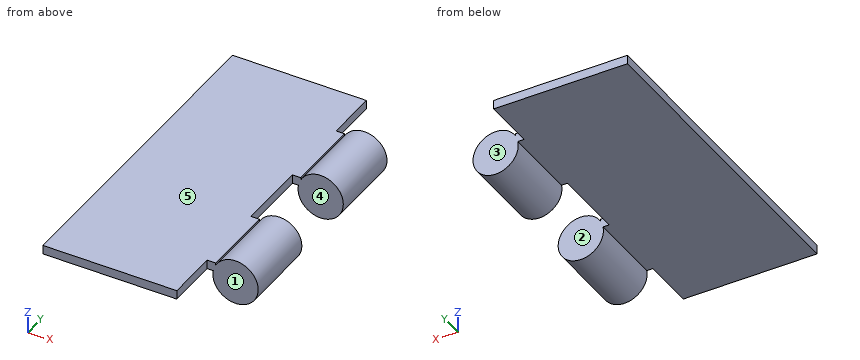
```python
from build123d import *

# Parameters (mm, degrees)
F0_W     = 31.1658
F0_H     = 76.073
F1_DEPTH = 2.0955
F2_W     = 17.526
F2_H     = 2.0955
F3_DEPTH = 1.9558
F4_R     = 5.2705
F5_DEPTH = 17.526
F7_DEPTH = 17.526


with BuildPart() as f1:
    # F0 (on Top) → F1 (new body)
    with BuildSketch(Plane.XY):
        Rectangle(F0_W, F0_H)
    extrude(amount=F1_DEPTH)

    # F2 (on face) → F3 (join)
    with BuildSketch(Plane.YZ.offset(15.5829)):
        with Locations((-17.0815, 1.04775)):
            Rectangle(F2_W, F2_H)
        with Locations((17.0815, 1.04775)):
            Rectangle(F2_W, F2_H)
    extrude(amount=F3_DEPTH)

    # F4 (on face) → F5 (join, through all)
    with BuildSketch(Plane.XZ.offset(25.8445)):
        with Locations((22.1742, -0.9652)):
            Circle(F4_R)
    extrude(amount=-F5_DEPTH)

    # F6 (on face) → F7 (join, through all)
    with BuildSketch(Plane.XZ.offset(-8.3185)):
        with BuildLine():
            Line((17.5387, 0), (16.992833, 0))
            ThreePointArc((16.992833, 0), (27.142883, -2.723141), (17.5387, 1.542849))
            Line((17.5387, 1.542849), (17.5387, 0))
        make_face()
    extrude(amount=-F7_DEPTH)


solid = f1.part
```
CAD build for the part. Positions are in the model's coordinates, mm. Face numbers are marked on the shaded views. A direction names the side the tool comes from. Round coordinates to 2 decimals unless told otherwise and drop trailing zeros. Order: outer loops, then holes, each group sorted by start corner. A loop starts at its lowest first (then second) coordinate and runs counter-clockwise, first axis right, second up. Notation, with made-up numbers: (37, 59.25) - (49, 59.25) arc R35 ccw to (49, 92.25) - close; hole circle Ø2 at (42, 88.25). An arc over 180 degrees is marked (long way). Answer as CSV lines item,"result". Start each with the question number.
1. Saw through at A-A, the plane z = -4.25. Write the cut outline in (x, y).
2. Tool access for the marked faces 1 and 2: list every direction of +Z, -Z, +X, -X, +Y, -Y with a clear straight run to the whole face (end or side of a thin tool).
3. Saw through at D-D, the plane x = 7. Write the cut outline in (y, z).
4. Pull direction Y, two halves, no side cores. Call the marked faces 3, 4 and 5: +Y half, -Y half, draft (parallel to the pull), parting line (faces both ways), or undercut.
5. Saw through at C-C, the plane x = 19.5. Write the cut outline in (y, z).
6. Pin check, flat tips, straight feed: pin 1 (5.5 mm diameter, centred on x = 21.5, z = -1, fed in from -Y); pin 2 (12 mm diameter, centred on x = -8.5, y = 20, fed in from +Z); pin 3 (1.5 mm diameter, centred on x = 18.5, z = 2.5, fed in from +Y); pin 4 (6 mm diameter, centred on x = -6, z = 2.5, fed in from -Y). Stop position of each tip, or through.
7. Saw through at B-B, the plane y = -21. Write the cut outline in (x, z), and give its area (3 significant figures).
8. Drill centre lines: L1, parallel to Y at x = 23, z = -1.25; L2, parallel to Z at x = -7.5, y = -11.5; L3, parallel to Z at x = 22.5, y = 22. Where is each one in solid material? Low to high. Write a range as [from, to].
Model answer:
1,outline,"(18.05, -25.84) - (26.3, -25.84) - (26.3, -8.32) - (18.05, -8.32) - close; (18.05, 8.32) - (26.3, 8.32) - (26.3, 25.84) - (18.05, 25.84) - close"
2,face 1,"+Z, -Z, +X, -Y"
2,face 2,"+Z, -Z, +X"
3,outline,"(-38.04, 0) - (38.04, 0) - (38.04, 2.1) - (-38.04, 2.1) - close"
4,face 3,"+Y half"
4,face 4,"undercut"
4,face 5,"draft"
5,outline,"(-25.84, -5.51) - (-8.32, -5.51) - (-8.32, 3.58) - (-25.84, 3.58) - close; (8.32, -5.51) - (25.84, -5.51) - (25.84, 3.58) - (8.32, 3.58) - close"
6,pin 1,"stops at y = -25.84"
6,pin 2,"stops at z = 2.1"
6,pin 3,"stops at y = 25.84"
6,pin 4,"stops at y = -38.04"
7,outline,"(-15.58, 0) - (16.99, 0) arc R5.27 ccw (long way) to (17.54, 1.54) - (17.54, 2.1) - (-15.58, 2.1) - close"
7,area,"156 mm²"
8,L1,"y = [-25.84, -8.32], [8.32, 25.84]"
8,L2,"z = [0, 2.1]"
8,L3,"z = [-6.23, 4.3]"
